Build history of the part. All positions in model axes, mm. A direction names the side the tool comes from. Round coordinates to 2 decimals unless told otherwise and drop trailing zeros. Write each loop counter-clockwise with the first axis right and the second up, starting at its lowest first coordinate (ties: lowest second). Pieces come first, ordered by that corner, then holes.
1) Saw through at A-A (x = 0). Write the cut outline in (y, z), plus the area to 3 significant figures.
2) Flat gauge pins, fed straight in: pin 1 (3 mm diameter, centred on y = 6, z = 1, fed in from +X); pin 2 (5 mm diameter, centred on x = 6, y = 12.5, fed in from -Z); pin 3 (1.5 mm diameter, centred on y = 14, z = -4, fed in from +X); pin 4 (3.5 mm diameter, centred on x = 0, z = 0, fed in from -Y). Where does each tip first touch, or does it go through?
3) Saw through at D-D (x = 5.25). Write the cut outline in (y, z), plus the area to 3 significant figures.
4) Saw through at B-B (z = 0). Write the cut outline in (x, y), plus the area to 3 significant figures.
5) Wall check: probe 1 along Z at (x, y) = (0, 10.25); probe 2 along X at (y, z) = (3.75, 0); probe 3 along Y at (x, z) = (7, 3.25). Give the ranges that are in metal, low to high.
6) Which spindle directions (+Z, -Z, +X, -X, +Y, -Y) get a long thin tool onto all of the face, cutting with end or side? Do faces 1 (the flat face through (-3.4, 0, 0.1)), 2 (the flat face through (6, 1, -2)). Say none if no direction does.
7) Saw through at C-C (y = 2.5). Write the cut outline in (x, z), plus the area to 3 significant figures.
8) Pull direction X, two halves, no side cores. Call faces 3 (the cylindrical face through (-3, 8, 0)), 4 (the flat face through (6, 8, -2)), 5 (the cylindrical face through (1.73, 0.49, 7.81)): +X half, -X half, draft (parallel to the pull), parting line (faces both ways), or undercut.
Autodesk Inventor part; units mm, degrees
ref_plane "YZ Plane" through (0, 0, 0) normal (1, 0, 0) x (0, 1, 0)
ref_plane "XZ Plane" through (0, 0, 0) normal (0, 1, 0) x (-1, 0, 0)
ref_plane "XY Plane" through (0, 0, 0) normal (0, 0, 1) x (1, 0, 0)
sketch "Boceto1" plane through (0, 0, 0) normal (0, 1, 0) x (-1, 0, 0)
  circle A0 centre (0, 0) radius 8
  dimension "d0" = 16
extrude "Extrusión1" add sketch "Boceto1" along normal blind 16
sketch "Boceto2" plane through (0, 16, 0) normal (0, 1, 0) x (1, 0, 0)
  circle A0 centre (0, 0) radius 3
  dimension "d3" = 6
extrude "Extrusión2" cut sketch "Boceto2" against normal blind 16
sketch "Boceto3" plane through (0, 0, 0) normal (1, 0, 0) x (0, 1, 0)
  line L0 (0, 8) -> (16, 8)
  line L1 (1, 8) -> (8, 8)
  line L2 (8, 8) -> (8, 6)
  line L3 (8, 6) -> (1, 6)
  line L4 (1, 6) -> (1, 8)
  line L5 (16, -8) -> (16, 8)
  line L6 (0, -8) -> (0, 8)
  line L7 (0, 0) -> (16, 0)
  dimension "d6" = 2
  dimension "d7" = 7
  dimension "d8" = 1
revolve "Revolución1" cut sketch "Boceto3" angle 360 about axis through (0, 0, 0) along (0, 1, 0) contours L0 L2 L3 L4
properties part number "20T pulley 6 mm bore GT2"
Evaluation:
1. outline: (0, -8) - (1, -8) - (1, -6) - (8, -6) - (8, -8) - (16, -8) - (16, -3) - (0, -3) - close; (0, 3) - (16, 3) - (16, 8) - (8, 8) - (8, 6) - (1, 6) - (1, 8) - (0, 8) - close
1. area: 132 mm2
2. pin 1: stops at x = 6
2. pin 2: stops at z = -7.19
2. pin 3: stops at x = 7.31
2. pin 4: passes through
3. outline: (0, -6.04) - (1, -6.04) - (1, -2.9) - (8, -2.9) - (8, -6.04) - (16, -6.04) - (16, 6.04) - (8, 6.04) - (8, 2.9) - (1, 2.9) - (1, 6.04) - (0, 6.04) - close
3. area: 149 mm2
4. outline: (-8, 0) - (-3, 0) - (-3, 16) - (-8, 16) - (-8, 8) - (-6, 8) - (-6, 1) - (-8, 1) - close; (3, 0) - (8, 0) - (8, 1) - (6, 1) - (6, 8) - (8, 8) - (8, 16) - (3, 16) - close
4. area: 132 mm2
5. probe 1: z = -8 to -3, 3 to 8
5. probe 2: x = -6 to -3, 3 to 6
5. probe 3: y = 0 to 1, 8 to 16
6. face 1: +Z, -Z, +X, -X, -Y
6. face 2: none
7. outline: circle Ø12 at (0, 0); hole circle Ø6 at (0, 0)
7. area: 84.8 mm2
8. face 3: undercut
8. face 4: draft
8. face 5: parting line
